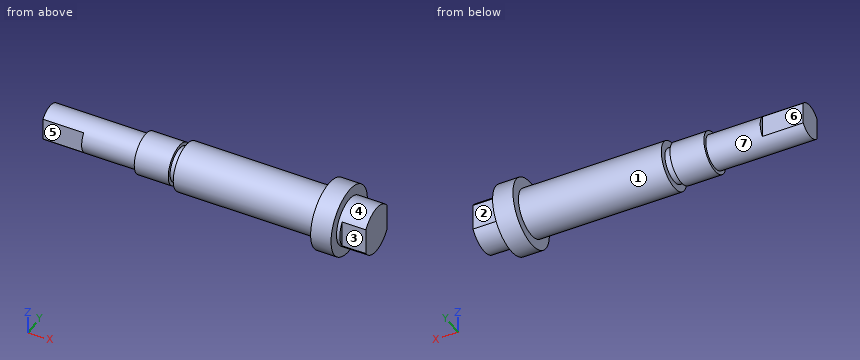
from build123d import *

# Parameters (mm, degrees)
SKETCH1_R           = 3.5
BOSS_EXTRUDE1_DEPTH = 50
BOSS_EXTRUDE2_START = 6
SKETCH2_R           = 5
BOSS_EXTRUDE2_DEPTH = 3
SKETCH5_R           = 3.5
SKETCH5_R_2         = 2.5
CUT_EXTRUDE2_DEPTH  = 20
BOSS_EXTRUDE3_START = 22
SKETCH3_R           = 3
BOSS_EXTRUDE3_DEPTH = 5
CUT_EXTRUDE3_START  = -5.5
CUT_EXTRUDE3_DEPTH  = 5.5
CUT_EXTRUDE4_START  = -2
CUT_EXTRUDE4_DEPTH  = 2
CUT_EXTRUDE5_DEPTH  = 6


with BuildPart() as part:
    # Sketch1 → Boss-Extrude1 (new body)
    with BuildSketch(Plane(origin=(0, 0, 0), x_dir=(0, 0, -1), z_dir=(1, 0, 0))):
        Circle(SKETCH1_R)
    extrude(amount=BOSS_EXTRUDE1_DEPTH)

    # Sketch2 → Boss-Extrude2 (add)
    with BuildSketch(Plane.ZY.offset(-50).offset(BOSS_EXTRUDE2_START)):
        Circle(SKETCH2_R)
    extrude(amount=BOSS_EXTRUDE2_DEPTH)

    # Sketch5 → Cut-Extrude2 (cut)
    with BuildSketch(Plane.ZY):
        Circle(SKETCH5_R)
        Circle(SKETCH5_R_2, mode=Mode.SUBTRACT)
    extrude(amount=-CUT_EXTRUDE2_DEPTH, mode=Mode.SUBTRACT)

    # Sketch3 → Boss-Extrude3 (add)
    with BuildSketch(Plane.ZY.offset(-41).offset(BOSS_EXTRUDE3_START)):
        Circle(SKETCH3_R)
    extrude(amount=BOSS_EXTRUDE3_DEPTH)

    # Sketch6 → Cut-Extrude3 (cut)
    with BuildSketch(Plane(origin=(50, 0, 0), x_dir=(0, 0, -1), z_dir=(1, 0, 0)).offset(CUT_EXTRUDE3_START)):
        with BuildLine():
            ThreePointArc((1.959591794, 2.9), (0, 3.5), (-1.959591794, 2.9))
            Line((-1.959591794, 2.9), (1.959591794, 2.9))
        make_face()
        with BuildLine():
            Line((1.959591794, -2.9), (-1.959591794, -2.9))
            ThreePointArc((-1.959591794, -2.9), (0, -3.5), (1.959591794, -2.9))
        make_face()
    extrude(amount=CUT_EXTRUDE3_DEPTH, mode=Mode.SUBTRACT)

    # Sketch7 → Cut-Extrude4 (cut)
    with BuildSketch(Plane(origin=(50, 0, 0), x_dir=(0, 0, -1), z_dir=(1, 0, 0)).offset(CUT_EXTRUDE4_START)):
        with BuildLine():
            Line((1.959591794, 2.9), (-1.959591794, 2.9))
            ThreePointArc((-1.959591794, 2.9), (-3.5, 0), (-1.959591794, -2.9))
            Line((-1.959591794, -2.9), (1.959591794, -2.9))
            ThreePointArc((1.959591794, -2.9), (3.5, 0), (1.959591794, 2.9))
        make_face()
    extrude(amount=CUT_EXTRUDE4_DEPTH, mode=Mode.SUBTRACT)

    # Sketch8 → Cut-Extrude5 (cut)
    with BuildSketch(Plane.ZY):
        with BuildLine():
            ThreePointArc((1.624807681, 1.9), (0, 2.5), (-1.624807681, 1.9))
            Line((-1.624807681, 1.9), (1.624807681, 1.9))
        make_face()
        with BuildLine():
            Line((1.624807681, -1.9), (-1.624807681, -1.9))
            ThreePointArc((-1.624807681, -1.9), (0, -2.5), (1.624807681, -1.9))
        make_face()
    extrude(amount=-CUT_EXTRUDE5_DEPTH, mode=Mode.SUBTRACT)


solid = part.part
Source: CAD feature listing. Evaluate the final solid. Frame: model axes, mm. Face numbers are marked on the shaded views. A direction names the side the tool comes from. Give positions to 0.01 mm unless a question says otherwise; leave off trailing zeros. Write each loop counter-clockwise with the first axis right and the second up, starting at its lowest first coordinate (ties: lowest second). Pieces come first, ordered by that corner, then holes. Notation, with made-up numbers: M 20,54.5 L 40,54.5 A14 ccw 40,66.5 Z; hole C 6.5,-22.5 d3. An arc over 180 degrees is marked long. Answer as a JSON object with one key per item and string values.
Q1. Ray query, line 1 along Z through (x, y) = (46.5, 0.25); line 2 along X through (y, z) = (4.75, -1.25); line 3 along X through (y, z) = (-2.5, 0.75). Return the intervals inside material, ascending.
Geometry check:
{"line 1": "z = -3.49 to 3.49", "line 2": "x = 41 to 44", "line 3": "x = 14 to 19, 20 to 48"}
Q2. Cut plane B-B, the plane y = 0. Return the cut outline in (x, z).
Geometry check:
{"outline": "M 0,-2.5 L 14,-2.5 L 14,-3 L 19,-3 L 19,-2.5 L 20,-2.5 L 20,-3.5 L 41,-3.5 L 41,-5 L 44,-5 L 44,-3.5 L 48,-3.5 L 48,3.5 L 44,3.5 L 44,5 L 41,5 L 41,3.5 L 20,3.5 L 20,2.5 L 19,2.5 L 19,3 L 14,3 L 14,2.5 L 0,2.5 Z"}
Q3. Mould query, pull axis Z, two halves, no side actions, for the marked faces 1 and 2. Classes: +Z half, -Z half, draft (parallel to the pull), parting line (faces both ways), or undercut.
Geometry check:
{"face 1": "parting line", "face 2": "draft"}
Q4. Access query for the marked faces 3, 4, 5, 6 and 7. Directions: +Z, -Z, +X, -X, +Y, -Y. A direction counts if a zero-diameter tool reaches every point of the face in a straight line with its end or side. Return the directions, or none.
Geometry check:
{"face 3": "+Z, -Z, +X, -Y", "face 4": "+X", "face 5": "+Z, -Z, -X, -Y", "face 6": "+Z, -Z, -X, +Y", "face 7": "-X"}
Q5. Contact query for flat-ended pins moving along their axis: P1, Ø2, axis at x = 19.5, z = 1.5, coming from the +Y side; P2, Ø1, axis at x = 47, z = 0.5, coming from the -Y side; P3, Ø3.5, axis at x = 1.5, z = 1, coming from the +Y side. Output: stop coordinate, or through.
Geometry check:
{"P1": "stops at y = 3.44", "P2": "stops at y = -2.9", "P3": "stops at y = 1.9"}
Q6. Cut plane C-C, the plane x = 5.5. Return the cut outline in (y, z).
Geometry check:
{"outline": "M -1.9,-1.62 A2.5 ccw 1.9,-1.62 L 1.9,1.62 A2.5 ccw -1.9,1.62 Z"}
Q7. Cut plane D-D, the plane x = 27. Return the cut outline in (y, z), then the cut area to 3 significant figures.
Geometry check:
{"outline": "C 0,0 d7", "area": "38.5 mm^2"}
